The model under review builds one solid part; all positions refer to its coordinate system, in mm. Face numbers are marked on the shaded views. A direction names the side the tool comes from. Give positions to 0.01 mm unless a question says otherwise; leave off trailing zeros. Write each loop counter-clockwise with the first axis right and the second up, starting at its lowest first coordinate (ties: lowest second). Pieces come first, ordered by that corner, then holes. Notation, with made-up numbers: (79.25, 60.5) - (117.25, 60.5) arc R14 ccw to (117.25, 77.5) - close; hole circle Ø8 at (-29.5, 10.5). An arc over 180 degrees is marked (long way). Write item = value, one per line.
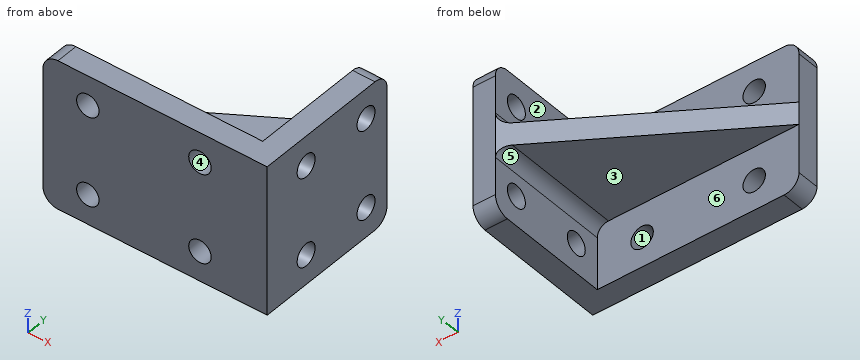
```python
from build123d import *

# Parameters (mm, degrees)
SKETCH_1_W           = 30
SKETCH_1_H           = 20
EXTRUDE_1_DEPTH      = 3
SKETCH_2_W           = 20
SKETCH_2_H           = 17
EXTRUDE_2_DEPTH      = 3
EXTRUDE_3_DEPTH      = 1.5
EXTRUDE_3_DEPTH_BACK = 1.5
SKETCH_4_R           = 1.5
CUT_EXTRUDE_1_DEPTH  = 40.862262856
SKETCH_5_R           = 1.5
CUT_EXTRUDE_2_DEPTH  = 40.102429592
FILLET_1_R           = 1.5
FILLET_2_R           = 2


with BuildPart() as part:
    # 草图1 → 凸台-拉伸1 (new body)
    with BuildSketch(Plane(origin=(0, 0, 0), x_dir=(1, 0, 0), z_dir=(0, 1, 0))):
        with Locations((15, 10)):
            Rectangle(SKETCH_1_W, SKETCH_1_H)
    extrude(amount=EXTRUDE_1_DEPTH)

    # 草图2 → 凸台-拉伸2 (add)
    with BuildSketch(Plane(origin=(30, 0, 0), x_dir=(0, 0, -1), z_dir=(1, 0, 0))):
        with Locations((10, 11.5)):
            Rectangle(SKETCH_2_W, SKETCH_2_H)
    extrude(amount=-EXTRUDE_2_DEPTH)

    # 草图3 → 凸台-拉伸3 (add, two sides: drawn at the far end of the back side and taken through both)
    with BuildSketch(Plane.XY.offset(-10).offset(-EXTRUDE_3_DEPTH_BACK)):
        Polygon((27, 20), (0, 3), (27, 3), align=None)
    extrude(amount=EXTRUDE_3_DEPTH + EXTRUDE_3_DEPTH_BACK)

    # 草图4 → 切除-拉伸1 (cut, through all)
    with BuildSketch(Plane(origin=(0, 3, 0), x_dir=(1, 0, 0), z_dir=(0, 1, 0))):
        with Locations(Location((6, 16, 0), (0, 0, 270))):
            Circle(SKETCH_4_R)
        with Locations(Location((21, 16, 0), (0, 0, 90))):
            Circle(SKETCH_4_R)
        with Locations(Location((21, 4, 0), (0, 0, 270))):
            Circle(SKETCH_4_R)
        with Locations(Location((6, 4, 0), (0, 0, 90))):
            Circle(SKETCH_4_R)
    extrude(amount=-CUT_EXTRUDE_1_DEPTH, mode=Mode.SUBTRACT)

    # 草图5 → 切除-拉伸2 (cut, through all)
    with BuildSketch(Plane.ZY.offset(-27)):
        with Locations((-16, 16.5)):
            Circle(SKETCH_5_R)
        with Locations(Location((-16, 6.5, 0), (0, 0, 180))):
            Circle(SKETCH_5_R)
        with Locations((-4, 6.5)):
            Circle(SKETCH_5_R)
        with Locations(Location((-4, 16.5, 0), (0, 0, 180))):
            Circle(SKETCH_5_R)
    extrude(amount=-CUT_EXTRUDE_2_DEPTH, mode=Mode.SUBTRACT)

    # 圆角1
    # the kernel refuses this fillet: 1.5 mm, written as the material it adds along each edge
    with BuildSketch(Plane(origin=(27, 3, -11.5), x_dir=(0, 0, -1), z_dir=(0, 1, 0))) as fillet_1_piece_1_section:
        with BuildLine():
            CenterArc((FILLET_1_R, FILLET_1_R), FILLET_1_R, 180, 90)
            Line((0, FILLET_1_R), (0, 0))
            Line((0, 0), (FILLET_1_R, 0))
        make_face()
    fillet_1_piece_1 = extrude(amount=20.75, mode=Mode.PRIVATE)
    fillet_1_piece_1 = split(fillet_1_piece_1, bisect_by=Plane(origin=(22.882537892, 17.407523858, -11.836797175), z_dir=(0.5328132696861393, -0.8462328400897506, 0)), keep=Keep.TOP, mode=Mode.PRIVATE)
    add(fillet_1_piece_1)
    with BuildSketch(Plane(origin=(27, -0.75, -8.5), x_dir=(0, 0, 1), z_dir=(0, 1, 0))) as fillet_1_piece_2_section:
        with BuildLine():
            CenterArc((FILLET_1_R, -FILLET_1_R), FILLET_1_R, 90, 90)
            Line((0, -FILLET_1_R), (0, 0))
            Line((0, 0), (FILLET_1_R, 0))
        make_face()
    fillet_1_piece_2 = extrude(amount=24.5, mode=Mode.PRIVATE)
    fillet_1_piece_2 = split(fillet_1_piece_2, bisect_by=Plane(origin=(26.667914796, 0, -8.163202825), z_dir=(0, 1, 0)), keep=Keep.TOP, mode=Mode.PRIVATE)
    fillet_1_piece_2 = split(fillet_1_piece_2, bisect_by=Plane(origin=(22.882537892, 17.407523858, -8.163202825), z_dir=(0.5328132696861393, -0.8462328400897506, 0)), keep=Keep.TOP, mode=Mode.PRIVATE)
    add(fillet_1_piece_2)

    # 圆角2
    fillet_2_edges = [part.edges().sort_by_distance(p)[0] for p in [
        (28.5, 20, 0),
        (28.5, 20, -20),
        (0, 1.5, -20),
        (0, 1.5, 0),
    ]]
    fillet(fillet_2_edges, radius=FILLET_2_R)


solid = part.part
```
1. Take a section at A-A on z = -4. Give the boundary of the cut face in (x, y), and give its area (3 significant figures).
Findings below:
outline = (0, 0) - (4.5, 0) - (4.5, 3) - (0, 3) - close; (7.5, 0) - (19.5, 0) - (19.5, 3) - (7.5, 3) - close; (22.5, 0) - (30, 0) - (30, 5) - (27, 5) - (27, 3) - (22.5, 3) - close; (27, 8) - (30, 8) - (30, 15) - (27, 15) - close; (27, 18) - (30, 18) - (30, 20) - (27, 20) - close
area = 105 mm²
2. Machinability: for the marked faces 1, 2 and 3, which of the approach directions +Z, -Z, +X, -X, +Y, -Y give a long, thin tool a straight path to every point of the face, cutting with its end or side? Answer none if there is none.
Findings below:
face_1 = +Y, -Y
face_2 = +Z, -X, +Y
face_3 = -Z, -X, +Y
3. Take a section at D-D on y = 6.5. Give the boundary of the cut face in (x, z), and give its area (3 significant figures).
Findings below:
outline = (5.56, -11.5) - (25.5, -11.5) arc R1.5 cw to (27, -13) - (27, -14.5) - (30, -14.5) - (30, -5.5) - (27, -5.5) - (27, -7) arc R1.5 cw to (25.5, -8.5) - (5.56, -8.5) - close; (27, -20) - (30, -20) - (30, -17.5) - (27, -17.5) - close; (27, -2.5) - (30, -2.5) - (30, 0) - (27, 0) - close
area = 107 mm²
4. Draft analysis for pull direction X (two halves, no side actions). For the marked faces 4, 5 and 6, state which applies: +X half, -X half, draft (parallel to the pull), parting line (faces both ways), or undercut.
Findings below:
face_4 = undercut
face_5 = -X half
face_6 = draft
5. For line 1 (X direction, y = 1.3, z = -16); line 2 (Y direction, x = 28.55, z = -16); line 3 (Z direction, x = 7, y = 2.75), list the stretches that pass through material, from the lowest coordinate up. Write a range as from..to.
Findings below:
line_1 = 0..4.5, 7.5..19.5, 22.5..30
line_2 = 0..5, 8..15, 18..20
line_3 = -20..-17.12, -14.88..-5.12, -2.88..0
6. Take a section at C-C on y = 2.25. Give the boundary of the cut face in (x, z), and give its area (3 significant figures).
Findings below:
outline = (0, -18) arc R2 ccw to (2, -20) - (30, -20) - (30, 0) - (2, 0) arc R2 ccw to (0, -2) - close; hole circle Ø3 at (6, -16); hole circle Ø3 at (6, -4); hole circle Ø3 at (21, -16); hole circle Ø3 at (21, -4)
area = 570 mm²
7. Take a section at B-B on x = 21. Give the boundary of the cut face in (y, z).
Findings below:
outline = (0, -20) - (3, -20) - (3, -17.5) - (0, -17.5) - close; (0, -14.5) - (3, -14.5) - (3, -11.5) - (16.22, -11.5) - (16.22, -8.5) - (3, -8.5) - (3, -5.5) - (0, -5.5) - close; (0, -2.5) - (3, -2.5) - (3, 0) - (0, 0) - close
8. Insertion check: P1, Ø7, axis at x = 7, z = -4.5, coming from the +Y side; P2, Ø2.5, axis at y = 6.5, z = -4, coming from the +X side; P3, Ø1.5, axis at x = 22, y = 6.5, coming from the -Z side; P4, Ø6, axis at x = 5, y = 7.5, coming from the +Z side. Each pin has a flat end and moves straight along its axis. Give the tip position at first contact, or say it passes through.
Findings below:
P1 = 3
P2 = through
P3 = -11.5
P4 = -8.5
